```python
from build123d import *

# Parameters (mm, degrees)
SKETCH_1_W          = 10
SKETCH_1_H          = 20
SKETCH_1_W_2        = 7.6
SKETCH_1_H_2        = 17.6
EXTRUDE_1_DEPTH     = 710
SKETCH_2_R          = 2.15
SKETCH_2_R_2        = 1.6
CUT_EXTRUDE_1_DEPTH = 711.299232718
SKETCH_3_R          = 2.15
SKETCH_3_R_2        = 1.6
CUT_EXTRUDE_2_DEPTH = 711.140831103
SKETCH_5_R          = 2.15
CUT_EXTRUDE_3_DEPTH = 711.140831103


with BuildPart() as part:
    # ｽｹｯﾁ1 → 押し出し-薄板1 (new body)
    with BuildSketch(Plane(origin=(0, 0, 0), x_dir=(0, 0, -1), z_dir=(1, 0, 0))):
        Rectangle(SKETCH_1_W, SKETCH_1_H)
        Rectangle(SKETCH_1_W_2, SKETCH_1_H_2, mode=Mode.SUBTRACT)
    extrude(amount=EXTRUDE_1_DEPTH)

    # ｽｹｯﾁ2 → ｶｯﾄ - 押し出し1 (cut, through all)
    with BuildSketch(Plane(origin=(0, 10, 0), x_dir=(1, 0, 0), z_dir=(0, 1, 0))):
        with Locations(Location((575, 0, 0), (0, 0, 270))):
            Circle(SKETCH_2_R)
        with Locations(Location((705, 0, 0), (0, 0, 270))):
            Circle(SKETCH_2_R)
        with Locations(Location((5, 0, 0), (0, 0, 270))):
            Circle(SKETCH_2_R)
        with Locations(Location((135, 0, 0), (0, 0, 270))):
            Circle(SKETCH_2_R)
        with Locations(Location((455, 0, 0), (0, 0, 270))):
            Circle(SKETCH_2_R)
        with Locations(Location((255, 0, 0), (0, 0, 270))):
            Circle(SKETCH_2_R)
        with Locations(Location((382.5, 0, 0), (0, 0, 270))):
            Circle(SKETCH_2_R_2)
        with Locations(Location((327.5, 0, 0), (0, 0, 270))):
            Circle(SKETCH_2_R_2)
    extrude(amount=-CUT_EXTRUDE_1_DEPTH, mode=Mode.SUBTRACT)

    # ｽｹｯﾁ3 → ｶｯﾄ - 押し出し2 (cut, through all)
    with BuildSketch(Plane.XY.offset(5)):
        with Locations((410, 5)):
            Circle(SKETCH_3_R)
        with Locations(Location((410, -5, 0), (0, 0, 90))):
            Circle(SKETCH_3_R)
        with Locations((690, 6)):
            Circle(SKETCH_3_R)
        with Locations(Location((690, -6, 0), (0, 0, 90))):
            Circle(SKETCH_3_R)
        with Locations(Location((20, 6, 0), (0, 0, 90))):
            Circle(SKETCH_3_R)
        with Locations((20, -6)):
            Circle(SKETCH_3_R)
        with Locations((300, -5)):
            Circle(SKETCH_3_R)
        with Locations(Location((300, 5, 0), (0, 0, 90))):
            Circle(SKETCH_3_R)
        with Locations((372.5, 0)):
            Circle(SKETCH_3_R_2)
        with Locations(Location((337.5, 0, 0), (0, 0, 90))):
            Circle(SKETCH_3_R_2)
        with Locations(Location((224.5, 5, 0), (0, 0, 90))):
            Circle(SKETCH_3_R)
        with Locations((110, 0)):
            Circle(SKETCH_3_R)
        with Locations((130, 0)):
            Circle(SKETCH_3_R)
        with Locations((150, 0)):
            Circle(SKETCH_3_R)
        with Locations(Location((560, 0, 0), (0, 0, 90))):
            Circle(SKETCH_3_R)
        with Locations(Location((580, 0, 0), (0, 0, 90))):
            Circle(SKETCH_3_R)
        with Locations(Location((600, 0, 0), (0, 0, 90))):
            Circle(SKETCH_3_R)
        with Locations((224.5, -5)):
            Circle(SKETCH_3_R)
        with Locations(Location((485.5, -5, 0), (0, 0, 90))):
            Circle(SKETCH_3_R)
        with Locations((485.5, 5)):
            Circle(SKETCH_3_R)
    extrude(amount=-CUT_EXTRUDE_2_DEPTH, mode=Mode.SUBTRACT)

    # ｽｹｯﾁ5 → ｶｯﾄ - 押し出し3 (cut, through all)
    with BuildSketch(Plane.XY.offset(5)):
        with Locations((380, 0)):
            Circle(SKETCH_5_R)
        with Locations(Location((330, 0, 0), (0, 0, 90))):
            Circle(SKETCH_5_R)
        with Locations((355, 0)):
            Circle(SKETCH_5_R)
    extrude(amount=-CUT_EXTRUDE_3_DEPTH, mode=Mode.SUBTRACT)


solid = part.part
```
Source: CAD feature listing. Evaluate the final solid. Frame: model axes, mm. Give positions to 0.01 mm unless a question says otherwise; leave off trailing zeros. Loops run counter-clockwise (first coordinate to the right, second up) from the corner with the lowest first, then second, coordinate; pieces in that order, holes last. Notation, with made-up numbers: (54, 37) -> (100, 37) arc R16 ccw to (100, 65) -> close; hole circle Ø5 at (0, 36). An arc over 180 degrees is marked (long way). Use a Markdown table: item, result. Add a question column.
(1) Section query B-B (z = 0). Count the separate pieces of the cut face and the enclosed holes in it, then the cut area to 3 significant figures.
(2) Ray query, line 1 (Y direction, x = 485.5, z = -4.5); line 2 (Z direction, x = 534, y = 7); line 3 (Y direction, x = 690, z = -4.6). Return the intervals inside material, ascending.
(3) First-contact query: pin 1 Ø4 at (x, z) = (5, 0) entering from +Y; pin 2 Ø5 at (x, y) = (20, 6) entering from -Z. Flat tips, straight axial feed; report the tip coordinate or a pass-through.
(4) Section query A-A (x = 364.5). Output: boundary loops of the cut face in (y, z).
(5) Pull-direction query (Z, two-part tool) for faces 1 (the face through (350, 0, 3.8)), 2 (the face through (350, 0, 5)), 3 (the face through (350, 0, -5)); classes: +Z half, -Z half, draft (parallel to the pull), parting line (faces both ways), or undercut.
Checked values:
| question | item | result |
|---|---|---|
| 1 | separate pieces | 18 |
| 1 | enclosed holes | 0 |
| 1 | area | 1,630 mm^2 |
| 2 | line 1 | -10 to -7.15, -2.85 to 2.85, 7.15 to 10 |
| 2 | line 2 | -5 to -3.8, 3.8 to 5 |
| 2 | line 3 | -10 to -8.15, -3.85 to 3.85, 8.15 to 10 |
| 3 | pin 1 | through |
| 3 | pin 2 | z = -5 |
| 4 | outline | (-10, -5) -> (10, -5) -> (10, 5) -> (-10, 5) -> close; hole (-8.8, -3.8) -> (8.8, -3.8) -> (8.8, 3.8) -> (-8.8, 3.8) -> close |
| 5 | face 1 | undercut |
| 5 | face 2 | +Z half |
| 5 | face 3 | -Z half |
